from build123d import *

# Parameters (mm, degrees)
CROQUIS1_W              = 4
CROQUIS1_H              = 5
CROQUIS1_R              = 1
SALIENTE_EXTRUIR1_DEPTH = 5
CROQUIS3_R              = 1.5
CORTAR_EXTRUIR1_DEPTH   = 1


with BuildPart() as part:
    # Croquis1 → Saliente-Extruir1 (new body)
    with BuildSketch(Plane.XY):
        Rectangle(CROQUIS1_W, CROQUIS1_H)
        Circle(CROQUIS1_R, mode=Mode.SUBTRACT)
    extrude(amount=SALIENTE_EXTRUIR1_DEPTH)

    # Croquis3 → Cortar-Extruir1 (cut)
    with BuildSketch(Plane(origin=(0, 2.5, 0), x_dir=(1, 0, 0), z_dir=(0, 1, 0))):
        with Locations((0, -2.5)):
            Circle(CROQUIS3_R)
    cortar_extruir1 = extrude(amount=-CORTAR_EXTRUIR1_DEPTH, mode=Mode.SUBTRACT)

    # Simetría1: Cortar-Extruir1 across plane
    add(cortar_extruir1.mirror(Plane(origin=(0, 0, 0), x_dir=(0, 0, 1), z_dir=(0, -1, 0))), mode=Mode.SUBTRACT)


solid = part.part
Model file for the job. Use its own axes, mm. A direction names the side the tool comes from. Give positions to 0.01 mm unless a question says otherwise; leave off trailing zeros. Order: outer loops, then holes, each group sorted by start corner. A loop starts at its lowest first (then second) coordinate and runs counter-clockwise, first axis right, second up. Notation, with made-up numbers: (16, 43.25) - (35, 43.25) arc R28 ccw to (35, 64.25) - close; hole circle Ø1 at (46, 29). An arc over 180 degrees is marked (long way). Write item = value, one per line. Start each with the question number.
1. Two-plate mould, pull along Y, no slides. Class faces 4 (the cylindrical face through (0, -1, 2)), 5 (the cylindrical face through (0, -2, 1)), 6 (the flat face through (0, -2.5, 0.8)), 7 (the flat face through (0, 2.5, 0.8)): pulls with the +Y half, pulls with the -Y half, needs draft (parallel to the pull), parting line crosses it, or undercut.
2. Cut at B-B, the plane x = 0. List the corners of the cut face in (y, z).
3. Cut at C-C, the plane z = 2.5. List the corners of the cut face in (x, y), and give its area (3 significant figures).
4. Drop a flat-ended pin along its axis: P1, Ø0.9, axis at x = -0.5, z = 3, coming from the +Y side. Give the stop position or say it passes through.
5. Cut at D-D, the plane x = 1.2. List the corners of the cut face in (y, z).
6. Cut at A-A, the plane y = 0. List the corners of the cut face in (x, z).
7. Which spindle directions (+Z, -Z, +X, -X, +Y, -Y) get a long thin tool onto all of the face, cutting with end or side? Do faces 1 (the flat face through (0, 1.5, 2)), 2 (the flat face through (0, -1.5, 2)), 3 (the flat face through (2, 0, 2)). Say none if no direction does.
8. Probe line 1 along X through (y, z) = (1.8, 2.5); line 2 along Z through (x, y) = (0, 2.1); line 3 along Y through (x, z) = (-0.05, 1.25). List the from-to ranges inside material, lowest first.
Taken from the geometry:
q1.face_4 = undercut
q1.face_5 = needs draft
q1.face_6 = pulls with the -Y half
q1.face_7 = pulls with the +Y half
q2.outline = (-2.5, 0) - (-1, 0) - (-1, 5) - (-2.5, 5) - (-2.5, 4) - (-1.5, 4) - (-1.5, 1) - (-2.5, 1) - close; (1, 0) - (2.5, 0) - (2.5, 1) - (1.5, 1) - (1.5, 4) - (2.5, 4) - (2.5, 5) - (1, 5) - close
q3.outline = (-2, -2.5) - (-1.5, -2.5) - (-1.5, -1.5) - (1.5, -1.5) - (1.5, -2.5) - (2, -2.5) - (2, 2.5) - (1.5, 2.5) - (1.5, 1.5) - (-1.5, 1.5) - (-1.5, 2.5) - (-2, 2.5) - close; hole circle Ø2 at (0, 0)
q3.area = 10.9 mm²
q4.P1 = 1.5
q5.outline = (-2.5, 0) - (2.5, 0) - (2.5, 1.6) - (1.5, 1.6) - (1.5, 3.4) - (2.5, 3.4) - (2.5, 5) - (-2.5, 5) - (-2.5, 3.4) - (-1.5, 3.4) - (-1.5, 1.6) - (-2.5, 1.6) - close
q6.outline = (-2, 0) - (-1, 0) - (-1, 5) - (-2, 5) - close; (1, 0) - (2, 0) - (2, 5) - (1, 5) - close
q7.face_1 = +Y
q7.face_2 = -Y
q7.face_3 = +Z, -Z, +X, +Y, -Y
q8.line_1 = -2 to -1.5, 1.5 to 2
q8.line_2 = 0 to 1, 4 to 5
q8.line_3 = -1.5 to -1, 1 to 1.5
